Read the model definition and answer for the solid it produces. Units are mm, in the model's axes. A direction names the side the tool comes from. Coordinates: 2 decimals unless noted, no trailing zeros. Loops run counter-clockwise (first coordinate to the right, second up) from the corner with the lowest first, then second, coordinate; pieces in that order, holes last. Notation, with made-up numbers: (45.25, 55.25) - (95.25, 55.25) arc R18 cw to (95.25, 75.25) - close; hole circle Ø2 at (47.5, -34.5). An arc over 180 degrees is marked (long way). Use one line per item in the form item = value.
from build123d import *

# Parameters (mm, degrees)
SKETCH_1_R      = 1.8
EXTRUDE_1_DEPTH = 32.5
FILLET_1_R      = 3


with BuildPart() as part:
    # 草图1 → 凸台-拉伸1 (new body)
    with BuildSketch(Plane(origin=(0, 0, 0), x_dir=(1, 0, 0), z_dir=(0, 1, 0))):
        Polygon((-67.5, 12.5), (-67.5, -12.5), (-47.5, -12.5), (-47.5, -5), (47.5, -5), (47.5, -12.5), (67.5, -12.5), (67.5, 12.5), (47.5, 12.5), (47.5, 5), (-47.5, 5), (-47.5, 12.5), align=None)
        with Locations(Location((-60, -9, 0), (0, 0, 270))):
            Circle(SKETCH_1_R, mode=Mode.SUBTRACT)
        with Locations(Location((60, -9, 0), (0, 0, 270))):
            Circle(SKETCH_1_R, mode=Mode.SUBTRACT)
        with Locations(Location((-60, 9, 0), (0, 0, 270))):
            Circle(SKETCH_1_R, mode=Mode.SUBTRACT)
        with Locations(Location((60, 9, 0), (0, 0, 270))):
            Circle(SKETCH_1_R, mode=Mode.SUBTRACT)
    extrude(amount=EXTRUDE_1_DEPTH)

    # 圆角1
    fillet_1_edges = [part.edges().sort_by_distance(p)[0] for p in [
        (47.5, 16.25, -12.5),
        (67.5, 16.25, -12.5),
        (67.5, 16.25, 12.5),
        (47.5, 16.25, 12.5),
        (47.5, 16.25, 5),
        (-47.5, 16.25, 5),
        (-47.5, 16.25, 12.5),
        (-67.5, 16.25, 12.5),
        (-67.5, 16.25, -12.5),
        (-47.5, 16.25, -12.5),
        (-47.5, 16.25, -5),
        (47.5, 16.25, -5),
    ]]
    fillet(fillet_1_edges, radius=FILLET_1_R)


solid = part.part
Item 1: For a pull along Z with two mould halves and no side action, classify faces 1 (the cylindrical face through (58.905, 16.022, 7.572)), 2 (the cylindrical face through (-58.215, 16.022, -9.234)), 3 (the cylindrical face through (-66.64, 16.48, -11.6)), 4 (the flat face through (-1, 32.5, 0)) as +Z half, -Z half, draft (parallel to the pull), parting line (faces both ways), or undercut.
Results below:
face_1 = undercut
face_2 = undercut
face_3 = -Z half
face_4 = draft
Item 2: The part is cut by section A-A on x = 60. Give the vertices of the cut face in (y, z).
Results below:
outline = (0, -12.5) - (32.5, -12.5) - (32.5, -10.8) - (0, -10.8) - close; (0, -7.2) - (32.5, -7.2) - (32.5, 7.2) - (0, 7.2) - close; (0, 10.8) - (32.5, 10.8) - (32.5, 12.5) - (0, 12.5) - close
Item 3: Each of these flat-tipped pins is pushed along its axis until it touches: P1, Ø4.5, axis at x = -60, z = 9, coming from the +Y side; P2, Ø5, axis at x = 19, y = 5, coming from the +Z side; P3, Ø16, axis at x = 3.5, y = 20, coming from the -Z side. Where does it stop, or does it pass through?
Results below:
P1 = 32.5
P2 = 5
P3 = -5
Item 4: Find the intervals of material crossed by L1, parallel to X at y = 9, z = -9; L2, parallel to X at y = 18.5, z = 9.5; L3, parallel to Z at x = -59.5, y = 22.5, in increasing order.
Results below:
L1 = -67.5 to -61.8, -58.2 to -47.5, 47.5 to 58.2, 61.8 to 67.5
L2 = -67.5 to -61.73, -58.27 to -47.5, 47.5 to 58.27, 61.73 to 67.5
L3 = -12.5 to -10.73, -7.27 to 7.27, 10.73 to 12.5
Item 5: Which of the six approach directions +Z, -Z, +X, -X, +Y, -Y give full straight-line access (tool end or side, diameter ignored) to faces 5 (the flat face through (-57, 16, -12.5)), 6 (the flat face through (-1, 16, 5)), 7 (the flat face through (1, 16, -5))?
Results below:
face_5 = -Z, +X, -X, +Y, -Y
face_6 = +Z, +Y, -Y
face_7 = -Z, +Y, -Y
Item 6: The part is cut by section B-B on y = 14. Give the vertices of the cut face in (x, z), plus the area to 3 significant figures.
Results below:
outline = (-67.5, -9.5) arc R3 ccw to (-64.5, -12.5) - (-50.5, -12.5) arc R3 ccw to (-47.5, -9.5) - (-47.5, -8) arc R3 cw to (-44.5, -5) - (44.5, -5) arc R3 cw to (47.5, -8) - (47.5, -9.5) arc R3 ccw to (50.5, -12.5) - (64.5, -12.5) arc R3 ccw to (67.5, -9.5) - (67.5, 9.5) arc R3 ccw to (64.5, 12.5) - (50.5, 12.5) arc R3 ccw to (47.5, 9.5) - (47.5, 8) arc R3 cw to (44.5, 5) - (-44.5, 5) arc R3 cw to (-47.5, 8) - (-47.5, 9.5) arc R3 ccw to (-50.5, 12.5) - (-64.5, 12.5) arc R3 ccw to (-67.5, 9.5) - close; hole circle Ø3.6 at (-60, -9); hole circle Ø3.6 at (-60, 9); hole circle Ø3.6 at (60, -9); hole circle Ø3.6 at (60, 9)
area = 1,900 mm²
Item 7: The part is cut by section C-C on x = 23. Give the vertices of the cut face in (y, z), plus the area to 3 significant figures.
Results below:
outline = (0, -5) - (32.5, -5) - (32.5, 5) - (0, 5) - close
area = 325 mm²
